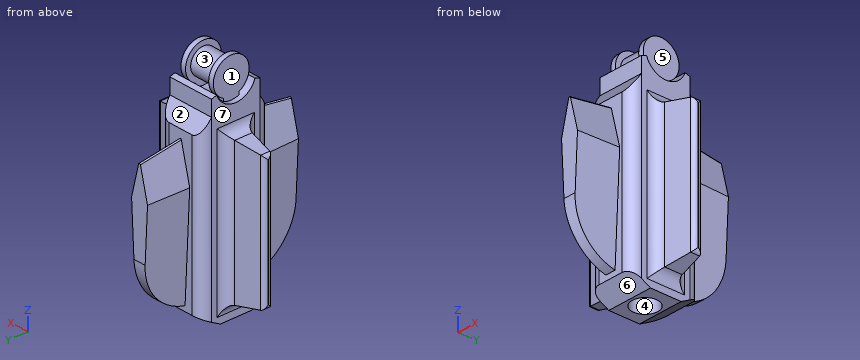
from build123d import *

# Parameters (mm, degrees)
SKETCH1_R                = 3.175
BOSS_EXTRUDE1_DEPTH      = 3.175
SKETCH2_R                = 4.445
BOSS_EXTRUDE2_DEPTH      = 1.27
SKETCH3_W                = 6.35
SKETCH3_H                = 3.81
BOSS_EXTRUDE3_DEPTH      = 1.27
BOSS_EXTRUDE4_DEPTH      = 8.89
BOSS_EXTRUDE4_DEPTH_BACK = 2.54
SKETCH5_R                = 3.175
CUT_EXTRUDE1_DEPTH       = 12.7
FILLET1_R                = 2.54
SKETCH6_W                = 35.56
SKETCH6_H                = 5.08
BOSS_EXTRUDE5_DEPTH      = 8.89
BOSS_EXTRUDE5_TAPER      = 10
FILLET2_R                = 1.016
FILLET3_R                = 2.54
BOSS_EXTRUDE6_DEPTH      = 10.16
BOSS_EXTRUDE6_TAPER      = 2
FILLET4_R                = 0.254
FILLET5_R                = 12.7


with BuildPart() as part:
    # Sketch1 → Boss-Extrude1 (new, symmetric)
    with BuildSketch(Plane(origin=(0, 0, 0), x_dir=(0, 0, -1), z_dir=(1, 0, 0))):
        Circle(SKETCH1_R)
    extrude(amount=BOSS_EXTRUDE1_DEPTH, both=True)

    # Sketch2 → Boss-Extrude2 (add)
    with BuildSketch(Plane(origin=(3.175, 0, 0), x_dir=(0, 0, -1), z_dir=(1, 0, 0))):
        Circle(SKETCH2_R)
    boss_extrude2 = extrude(amount=BOSS_EXTRUDE2_DEPTH)

    # Mirror1: Boss-Extrude2 across plane
    add(boss_extrude2.mirror(Plane(origin=(0, 0, 0), x_dir=(0, 0, 1), z_dir=(1, 0, 0))))

    # Sketch3 → Boss-Extrude3 (add)
    with BuildSketch(Plane(origin=(4.445, 0, 0), x_dir=(0, 0, -1), z_dir=(1, 0, 0))):
        with Locations((3.175, 0)):
            Rectangle(SKETCH3_W, SKETCH3_H)
    boss_extrude3 = extrude(amount=-BOSS_EXTRUDE3_DEPTH)

    # Mirror2: Boss-Extrude3 across plane
    add(boss_extrude3.mirror(Plane(origin=(0, 0, 0), x_dir=(0, 0, 1), z_dir=(1, 0, 0))))

    # Sketch4 → Boss-Extrude4 (add, two sides: drawn at the far end of the back side and taken through both)
    with BuildSketch(Plane(origin=(-3.175, 0, 0), x_dir=(0, 0, -1), z_dir=(1, 0, 0)).offset(-BOSS_EXTRUDE4_DEPTH_BACK)):
        with BuildLine():
            Line((1.737462328, 4.773638514), (2.118462328, 6.043638514))
            Line((2.118462328, 6.043638514), (5.928462328, 6.043638514))
            Line((5.928462328, 6.043638514), (9.738462328, 8.583638514))
            Line((9.738462328, 8.583638514), (47.838462328, 8.583638514))
            Line((47.838462328, 8.583638514), (50.378462328, 3.81))
            Line((50.378462328, 3.81), (50.378462328, -3.81))
            Line((50.378462328, -3.81), (47.838462328, -8.583638514))
            Line((47.838462328, -8.583638514), (9.738462328, -8.583638514))
            Line((9.738462328, -8.583638514), (5.928462328, -6.043638514))
            Line((5.928462328, -6.043638514), (2.118462328, -6.043638514))
            Line((2.118462328, -6.043638514), (1.737462328, -4.773638514))
            ThreePointArc((1.737462328, -4.773638514), (5.08, 0), (1.737462328, 4.773638514))
        make_face()
    extrude(amount=BOSS_EXTRUDE4_DEPTH + BOSS_EXTRUDE4_DEPTH_BACK)

    # Sketch5 → Cut-Extrude1 (cut)
    with BuildSketch(Plane(origin=(0, 0, -50.378462328), x_dir=(-1, 0, 0), z_dir=(0, 0, -1))):
        Circle(SKETCH5_R)
    extrude(amount=-CUT_EXTRUDE1_DEPTH, mode=Mode.SUBTRACT)

    # Fillet1
    fillet1_edges = [part.edges().sort_by_distance(p)[0] for p in [
        (5.715, -8.583638514, -28.788462328),
        (-5.715, -8.583638514, -28.788462328),
        (-5.715, 8.583638514, -28.788462328),
        (5.715, 8.583638514, -28.788462328),
    ]]
    fillet(fillet1_edges, radius=FILLET1_R)

    # Sketch6 → Boss-Extrude5 (add)
    with BuildSketch(Plane(origin=(5.715, 0, 0), x_dir=(0, 0, -1), z_dir=(1, 0, 0))):
        with Locations((28.788462328, 0)):
            Rectangle(SKETCH6_W, SKETCH6_H)
    boss_extrude5 = extrude(amount=BOSS_EXTRUDE5_DEPTH, taper=BOSS_EXTRUDE5_TAPER)

    # Mirror3: Boss-Extrude5 across plane
    add(boss_extrude5.mirror(Plane(origin=(0, 0, 0), x_dir=(0, 0, 1), z_dir=(1, 0, 0))))

    # Fillet2
    fillet2_edges = [part.edges().sort_by_distance(p)[0] for p in [
        (14.605, 0, -12.576009187),
        (14.605, -0.972453142, -28.788462328),
        (14.605, 0, -45.00091547),
        (14.605, 0.972453142, -28.788462328),
        (-14.605, 0, -12.576009187),
        (-14.605, 0.972453142, -28.788462328),
        (-14.605, 0, -45.00091547),
        (-14.605, -0.972453142, -28.788462328),
    ]]
    fillet(fillet2_edges, radius=FILLET2_R)

    # Fillet3
    fillet3_edges = [part.edges().sort_by_distance(p)[0] for p in [
        (5.715, 0, -11.008462328),
        (5.715, -2.54, -28.788462328),
        (5.715, 0, -46.568462328),
        (5.715, 2.54, -28.788462328),
        (-5.715, 0, -11.008462328),
        (-5.715, -2.54, -28.788462328),
        (-5.715, 0, -46.568462328),
        (-5.715, 2.54, -28.788462328),
    ]]
    fillet(fillet3_edges, radius=FILLET3_R)

    # Sketch7 → Boss-Extrude6 (add)
    with BuildSketch(Plane(origin=(0, 8.583638514, 0), x_dir=(1, 0, 0), z_dir=(0, 1, 0))):
        Polygon((-1.27, 46.568462328), (-2.54, 21.168462328), (0, 11.008462328), (2.54, 21.168462328), (1.27, 46.568462328), align=None)
    boss_extrude6 = extrude(amount=BOSS_EXTRUDE6_DEPTH, taper=BOSS_EXTRUDE6_TAPER)

    # Mirror4: Boss-Extrude6 across plane
    add(boss_extrude6.mirror(Plane.ZX))

    # Fillet4
    fillet4_edges = [part.edges().sort_by_distance(p)[0] for p in [
        (0, 13.663638514, -11.739890995),
        (0, -13.663638514, -11.739890995),
    ]]
    fillet(fillet4_edges, radius=FILLET4_R)

    # Fillet5
    # the kernel refuses this fillet: 12.7 mm, written as the material it takes off along each edge
    with BuildSketch(Plane(origin=(31.154033704, -18.743638514, -46.21366731), x_dir=(0, 0.9993908270191081, -0.034899496702148744), z_dir=(-1, 0, 0))) as fillet5_piece_1:
        with BuildLine():
            CenterArc((12.270376998, -12.524472427), FILLET5_R, 99.536959033, 78.463040967)
            Line((-0.421886505, -12.081248819), (-0.675731775, -12.072384347))
            Line((-0.675731775, -12.072384347), (-0.25384527, 0.008864472))
            Line((-0.25384527, 0.008864472), (0, 0.254))
            ThreePointArc((0, 0.254), (5.083096485, 0.254), (10.12410929, 0.250489449))
            Line((10.12410929, 0.250489449), (10.16619297, 0))
        make_face()
    extrude(amount=62.308067408, mode=Mode.SUBTRACT)
    with BuildSketch(Plane(origin=(31.154033704, 18.743638514, -46.21366731), x_dir=(0, -0.9993908270191081, -0.034899496702148744), z_dir=(-1, 0, 0))) as fillet5_piece_2:
        with BuildLine():
            CenterArc((12.270376998, 12.524472427), FILLET5_R, 182, 78.463040967)
            Line((-0.421886505, 12.081248819), (-0.675731775, 12.072384347))
            Line((-0.675731775, 12.072384347), (-0.25384527, -0.008864472))
            Line((-0.25384527, -0.008864472), (0, -0.254))
            ThreePointArc((0, -0.254), (5.083096485, -0.254), (10.12410929, -0.250489449))
            Line((10.12410929, -0.250489449), (10.16619297, 0))
        make_face()
    extrude(amount=62.308067408, mode=Mode.SUBTRACT)


solid = part.part
Could you check a few things on this model? Use its own coordinates, in mm. Face numbers are marked on the shaded views. A direction names the side the tool comes from. Give positions to 0.01 mm unless a question says otherwise; leave off trailing zeros. Order: outer loops, then holes, each group sorted by start corner. A loop starts at its lowest first (then second) coordinate and runs counter-clockwise, first axis right, second up.
1. Thinking about a two-plate mould opening in Y: for the marked faces 5, 6 and 7, which applies, +Y half, -Y half, draft (parallel to the pull), parting line (faces both ways), or undercut?
Answers below:
face 5: undercut
face 6: -Y half
face 7: draft
2. Suppose I cut it at A-A (z = 0). Write out the boundary of the cut face in (x, y) (3 decimals).
Answers below:
outline: (-4.445, -4.445) - (-3.175, -4.445) - (-3.175, -3.175) - (3.175, -3.175) - (3.175, -4.445) - (4.445, -4.445) - (4.445, 4.445) - (3.175, 4.445) - (3.175, 3.175) - (-3.175, 3.175) - (-3.175, 4.445) - (-4.445, 4.445) - close
3. Which directions (+Z, -Z, +X, -X, +Y, -Y) give clear straight access to the entire face, cutting with the end or side of a thin tool? Please do the marked faces 1, 2, 3 and 4.
Answers below:
face 1: +Z, -X
face 2: +Z, +X, -X, +Y
face 3: none
face 4: -Z
4. For pin 1 (1.9 mm diameter, centred on x = -0.5, z = -38, fed in from -Y); pin 2 (8 mm diameter, centred on x = 10.5, z = -19.5, fed in from -Y); pin 3 (5 mm diameter, centred on x = -1, z = -7.5, fed in from +Y); pin 4 (1 mm diameter, centred on y = -10, z = -7.5, fed in from -X), each with a flat end and sliding along its axis, tell me the tip position at first contact or that it passes through.
Answers below:
pin 1: stops at y = -18.4
pin 2: stops at y = -2.84
pin 3: stops at y = 8.58
pin 4: passes through
5. I need wall thicknesses on L1, parallel to Y at x = 5, z = -44; L2, parallel to X at y = 1.5, z = 2.5 (3 decimals); L3, parallel to Z at x = -1.25, y = 1. Which ranges of each line are inside material? Lowest first, please.
Answers below:
L1: y = -7.81 to 7.81
L2: x = -4.445 to 4.445
L3: z = -37.68 to -4.98, -3.01 to 3.01
